from build123d import *

# Parameters (mm, degrees)
ESQUISSE1_R        = 1.5
ESQUISSE1_W        = 5
ESQUISSE1_H        = 5
BOSS_EXTRU_1_DEPTH = 5


with BuildPart() as part:
    # Esquisse1 → Boss.-Extru.1 (new body)
    with BuildSketch(Plane.XY):
        with BuildLine():
            ThreePointArc((-55.961524227, -23.07179677), (-58.889727457, -34), (-47.961524227, -36.92820323))
            ThreePointArc((-47.961524227, -36.92820323), (0, -30.420831874), (47.961524227, -36.92820323))
            ThreePointArc((47.961524227, -36.92820323), (58.889727457, -34), (55.961524227, -23.07179677))
            ThreePointArc((55.961524227, -23.07179677), (26.345213207, 15.210415937), (8, 60))
            ThreePointArc((8, 60), (0, 68), (-8, 60))
            ThreePointArc((-8, 60), (-26.345213207, 15.210415937), (-55.961524227, -23.07179677))
        make_face()
        with Locations((43.301270189, -25)):
            Circle(ESQUISSE1_R, mode=Mode.SUBTRACT)
        with Locations((0, 50)):
            Circle(ESQUISSE1_R, mode=Mode.SUBTRACT)
        with Locations((-43.301270189, -25)):
            Circle(ESQUISSE1_R, mode=Mode.SUBTRACT)
        with BuildLine():
            Line((2.7, 21.833689565), (4.179128531, 21.59941862))
            ThreePointArc((4.179128531, 21.59941862), (7.58132701, 23.332925329), (9.314833719, 19.93072685))
            Line((9.314833719, 19.93072685), (10.649174844, 19.250846089))
            ThreePointArc((10.649174844, 19.250846089), (14.42054091, 19.848171792), (15.017866614, 16.076805726))
            Line((15.017866614, 16.076805726), (16.076805726, 15.017866614))
            ThreePointArc((16.076805726, 15.017866614), (19.848171792, 14.42054091), (19.250846089, 10.649174844))
            Line((19.250846089, 10.649174844), (19.93072685, 9.314833719))
            ThreePointArc((19.93072685, 9.314833719), (23.332925329, 7.58132701), (21.59941862, 4.179128531))
            Line((21.59941862, 4.179128531), (21.833689565, 2.7))
            ThreePointArc((21.833689565, 2.7), (24.533689565, 0), (21.833689565, -2.7))
            Line((21.833689565, -2.7), (21.59941862, -4.179128531))
            ThreePointArc((21.59941862, -4.179128531), (23.332925329, -7.58132701), (19.93072685, -9.314833719))
            Line((19.93072685, -9.314833719), (19.250846089, -10.649174844))
            ThreePointArc((19.250846089, -10.649174844), (19.848171792, -14.42054091), (16.076805726, -15.017866614))
            Line((16.076805726, -15.017866614), (15.017866614, -16.076805726))
            ThreePointArc((15.017866614, -16.076805726), (14.42054091, -19.848171792), (10.649174844, -19.250846089))
            Line((10.649174844, -19.250846089), (9.314833719, -19.93072685))
            ThreePointArc((9.314833719, -19.93072685), (7.58132701, -23.332925329), (4.179128531, -21.59941862))
            Line((4.179128531, -21.59941862), (2.7, -21.833689565))
            ThreePointArc((2.7, -21.833689565), (0, -24.533689565), (-2.7, -21.833689565))
            Line((-2.7, -21.833689565), (-4.179128531, -21.59941862))
            ThreePointArc((-4.179128531, -21.59941862), (-7.58132701, -23.332925329), (-9.314833719, -19.93072685))
            Line((-9.314833719, -19.93072685), (-10.649174844, -19.250846089))
            ThreePointArc((-10.649174844, -19.250846089), (-14.42054091, -19.848171792), (-15.017866614, -16.076805726))
            Line((-15.017866614, -16.076805726), (-16.076805726, -15.017866614))
            ThreePointArc((-16.076805726, -15.017866614), (-19.848171792, -14.42054091), (-19.250846089, -10.649174844))
            Line((-19.250846089, -10.649174844), (-19.93072685, -9.314833719))
            ThreePointArc((-19.93072685, -9.314833719), (-23.332925329, -7.58132701), (-21.59941862, -4.179128531))
            Line((-21.59941862, -4.179128531), (-21.833689565, -2.7))
            ThreePointArc((-21.833689565, -2.7), (-24.533689565, 0), (-21.833689565, 2.7))
            Line((-21.833689565, 2.7), (-21.59941862, 4.179128531))
            ThreePointArc((-21.59941862, 4.179128531), (-23.332925329, 7.58132701), (-19.93072685, 9.314833719))
            Line((-19.93072685, 9.314833719), (-19.250846089, 10.649174844))
            ThreePointArc((-19.250846089, 10.649174844), (-19.848171792, 14.42054091), (-16.076805726, 15.017866614))
            Line((-16.076805726, 15.017866614), (-15.017866614, 16.076805726))
            ThreePointArc((-15.017866614, 16.076805726), (-14.42054091, 19.848171792), (-10.649174844, 19.250846089))
            Line((-10.649174844, 19.250846089), (-9.314833719, 19.93072685))
            ThreePointArc((-9.314833719, 19.93072685), (-7.58132701, 23.332925329), (-4.179128531, 21.59941862))
            Line((-4.179128531, 21.59941862), (-2.7, 21.833689565))
            ThreePointArc((-2.7, 21.833689565), (0, 24.533689565), (2.7, 21.833689565))
        make_face(mode=Mode.SUBTRACT)
        Polygon((40.22114317, -20.334936491), (35.891016151, -17.834936491), (33.391016151, -22.165063509), (37.72114317, -24.665063509), align=None, mode=Mode.SUBTRACT)
        Polygon((48.881397208, -25.334936491), (53.211524227, -27.834936491), (50.711524227, -32.165063509), (46.381397208, -29.665063509), align=None, mode=Mode.SUBTRACT)
        with Locations((0, 57.5)):
            Rectangle(ESQUISSE1_W, ESQUISSE1_H, mode=Mode.SUBTRACT)
        with Locations((0, 42.5)):
            Rectangle(ESQUISSE1_W, ESQUISSE1_H, mode=Mode.SUBTRACT)
        Polygon((-48.881397208, -25.334936491), (-53.211524227, -27.834936491), (-50.711524227, -32.165063509), (-46.381397208, -29.665063509), align=None, mode=Mode.SUBTRACT)
        Polygon((-40.22114317, -20.334936491), (-35.891016151, -17.834936491), (-33.391016151, -22.165063509), (-37.72114317, -24.665063509), align=None, mode=Mode.SUBTRACT)
    extrude(amount=BOSS_EXTRU_1_DEPTH)


solid = part.part
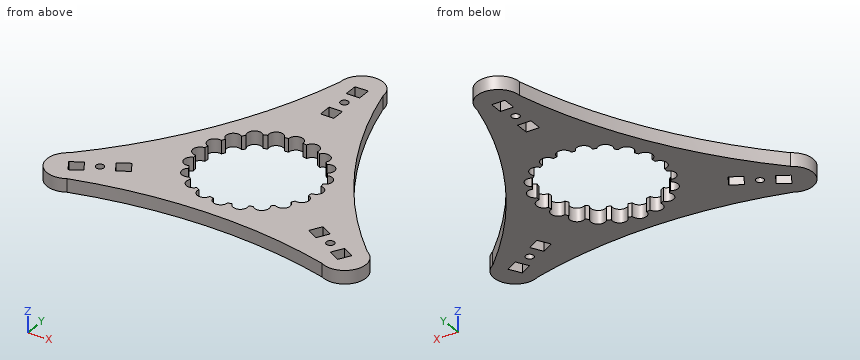
Build history of the part. All positions in model axes, mm. Round coordinates to 2 decimals unless told otherwise and drop trailing zeros. Write each loop counter-clockwise with the first axis right and the second up, starting at its lowest first coordinate (ties: lowest second). Pieces come first, ordered by that corner, then holes. Notation, with made-up numbers: M 46,-35.75 L 65,-35.75 A22 cw 65,-12.75 Z; hole C -38,1.25 d9. An arc over 180 degrees is marked long. Answer in a Markdown table with one row per item.
1. Flat gauge pins, fed straight in: P1, Ø3.5, axis at x = 43.3, y = -25, coming from the -Z side; P2, Ø3, axis at y = 29, z = 2, coming from the +X side; P3, Ø1, axis at x = 29, z = 3.5, coming from the +Y side; P4, Ø2.5, axis at x = -43.3, y = -25, coming from the +Z side. Where does each tip first touch, or does it go through?
Geometry check:
| item | result |
|---|---|
| P1 | z = 0 |
| P2 | x = 19.87 |
| P3 | y = 11.58 |
| P4 | through |
2. Saw through at C-C (z = 2.6). State how many separate pieces and enclosed holes the cut face has, and give its area (3 significant figures).
Geometry check:
| item | result |
|---|---|
| separate pieces | 1 |
| enclosed holes | 10 |
| area | 3,890 mm2 |
3. Saw through at A-A (x = 0). List the corners of the cut face in (y, z).
Geometry check:
| item | result |
|---|---|
| outline | M -30.42,0 L -24.53,0 L -24.53,5 L -30.42,5 Z; M 24.53,0 L 40,0 L 40,5 L 24.53,5 Z; M 45,0 L 48.5,0 L 48.5,5 L 45,5 Z; M 51.5,0 L 55,0 L 55,5 L 51.5,5 Z; M 60,0 L 68,0 L 68,5 L 60,5 Z |
4. Saw through at D-D (y = 50). List the corners of the cut face in (x, z), and give its area (3 significant figures).
Geometry check:
| item | result |
|---|---|
| outline | M -10.91,0 L -1.5,0 L -1.5,5 L -10.91,5 Z; M 1.5,0 L 10.91,0 L 10.91,5 L 1.5,5 Z |
| area | 94.1 mm2 |
5. Probe L1, parallel to X at y = -27, z = 4.45; L2, parallel to X at y = -18, z = 3.35; L3, parallel to Y at x = 35.5, z = 1.7. List the from-to ranges inside material, lowest first. Write a range as [from, to].
Geometry check:
| item | result |
|---|---|
| L1 | [-59.38, -51.77], [-47.92, 47.92], [51.77, 59.38] |
| L2 | [-51.01, -36.18], [-35.8, -15.51], [15.51, 35.8], [36.18, 51.01] |
| L3 | [-33.96, -23.38], [-18.51, 0.95] |
6. Saw through at B-B (y = 0). List the corners of the cut face in (x, z), and give its area (3 significant figures).
Geometry check:
| item | result |
|---|---|
| outline | M -36.18,0 L -24.53,0 L -24.53,5 L -36.18,5 Z; M 24.53,0 L 36.18,0 L 36.18,5 L 24.53,5 Z |
| area | 116 mm2 |
